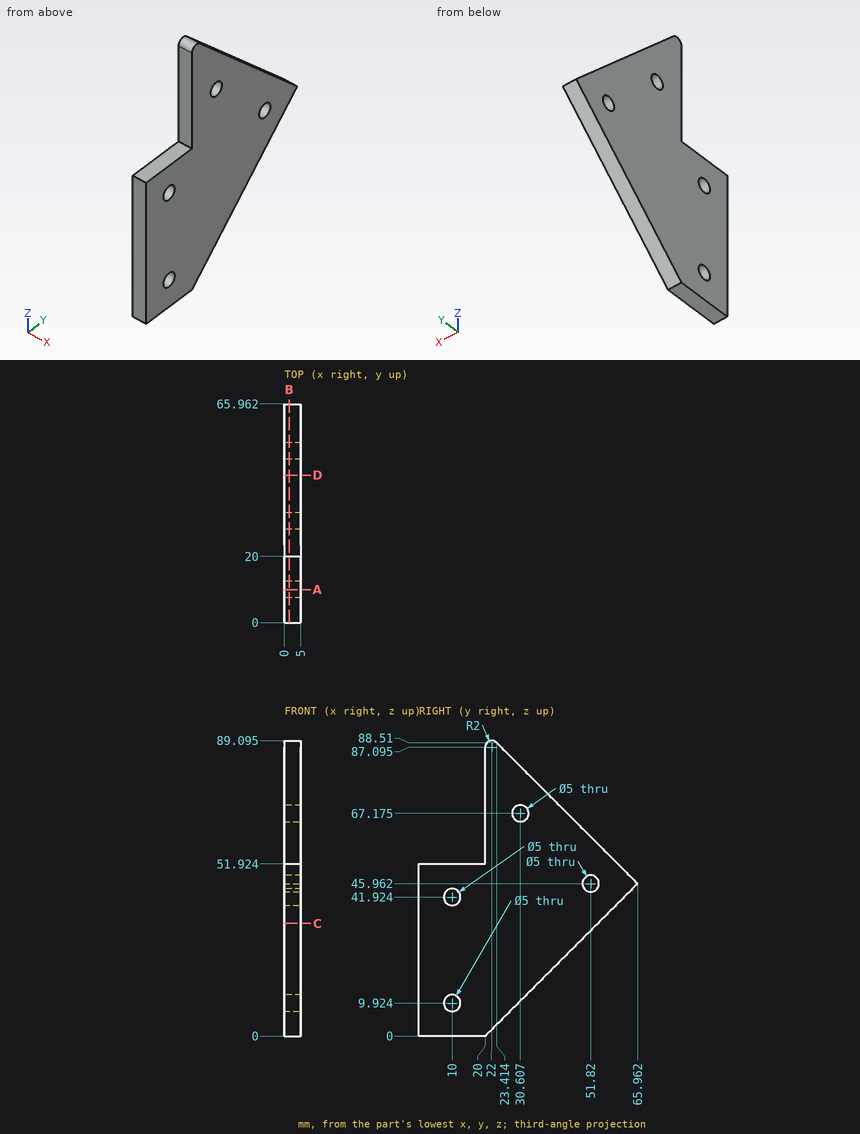
Here's the drawing with two shaded views (mm, measured from the low corner). I have some questions. Round coordinates to 2 decimals unless told otherwise and drop trailing zeros. Order: outer loops, then holes, each group sorted by start corner. A loop starts at its lowest first (then second) coordinate and runs counter-clockwise, first axis right, second up. Notation, with made-up numbers: (11, 77) -> (24, 77) arc R11 cw to (24, 94) -> close; hole circle Ø9 at (7, -21). An arc over 180 degrees is marked (long way). Return JSON: item names as keys, results as strings.
Q1. If we section it at C-C on z = 34: List the corners of the cut face in (x, y) for me.
Filled sheet:
{"outline": "(0, 0) -> (5, 0) -> (5, 54) -> (0, 54) -> close"}
Q2. I need wall thicknesses on line 1 along Z through (x, y) = (4, 4); line 2 along Y through (x, z) = (1.5, 9) (1 decimal); line 3 along Z through (x, y) = (1.2, 9.5) (1 decimal). Which ranges of each line are inside material? Lowest first, please. Write a range as from..to.
Filled sheet:
{"line 1": "z = 0..51.92", "line 2": "y = 0..7.7, 12.3..29", "line 3": "z = 0..7.5, 12.4..39.5, 44.4..51.9"}
Q3. If we section it at A-A on y = 10: List the corners of the cut face in (x, z) for me, plus the area to 3 significant figures.
Filled sheet:
{"outline": "(0, 0) -> (5, 0) -> (5, 7.42) -> (0, 7.42) -> close; (0, 12.42) -> (5, 12.42) -> (5, 39.42) -> (0, 39.42) -> close; (0, 44.42) -> (5, 44.42) -> (5, 51.92) -> (0, 51.92) -> close", "area": "210 mm^2"}
Q4. If we section it at D-D on y = 44.5: List the corners of the cut face in (x, z) for me.
Filled sheet:
{"outline": "(0, 24.5) -> (5, 24.5) -> (5, 67.42) -> (0, 67.42) -> close"}
Q5. If we section it at B-B on x = 1.45: List the corners of the cut face in (y, z) for me (1 decimal).
Filled sheet:
{"outline": "(0, 0) -> (20, 0) -> (66, 46) -> (23.4, 88.5) arc R2 ccw to (20, 87.1) -> (20, 51.9) -> (0, 51.9) -> close; hole circle Ø5 at (10, 9.9); hole circle Ø5 at (10, 41.9); hole circle Ø5 at (30.6, 67.2); hole circle Ø5 at (51.8, 46)"}
Q6. For pin 1 Ø1 at (x, z) = (1, 10.5) entering from +Y; pin 2 Ø4 at (y, z) = (51.82, 45.96) entering from +X; pin 3 Ø1.5 at (x, y) = (3.5, 11.5) entering from +Z; pin 4 Ø1 at (x, y) = (0.5, 43) entering from +Z (1 decimal), each with a flat end and sliding along its axis, tell me the tip position at first contact or that it passes through.
Filled sheet:
{"pin 1": "stops at y = 31", "pin 2": "passes through", "pin 3": "stops at z = 51.92", "pin 4": "stops at z = 69.4"}
